```python
from build123d import *

# Parameters (mm, degrees)
ESQUISSE1_W             = 22.5
ESQUISSE1_H             = 80
BOSS_EXTRU_1_DEPTH      = 3
ESQUISSE2_W             = 3
ESQUISSE2_H             = 80
BOSS_EXTRU_2_DEPTH      = 111.5
ESQUISSE3_W             = 22.5
ESQUISSE3_H             = 80
BOSS_EXTRU_3_DEPTH      = 3
ESQUISSE4_R             = 5.25
ENL_V_MAT_EXTRU_1_DEPTH = 2.2
ENL_V_START             = -1.8
ENL_V_MAT_EXTRU_2_DEPTH = 1.2
ENL_V_START_2           = -2.2
ESQUISSE6_R             = 5.25
ENL_V_MAT_EXTRU_3_DEPTH = 2.2
BOSS_EXTRU_4_DEPTH      = 1
ESQUISSE8_R             = 1.6
ENL_V_MAT_EXTRU_4_DEPTH = 4
CONG_2_R                = 1


with BuildPart() as part:
    # Esquisse1 → Boss.-Extru.1 (new body)
    with BuildSketch(Plane.XY):
        with Locations((11.25, 40)):
            Rectangle(ESQUISSE1_W, ESQUISSE1_H)
    extrude(amount=BOSS_EXTRU_1_DEPTH)

    # Esquisse2 → Boss.-Extru.2 (add)
    with BuildSketch(Plane.XY.offset(3)):
        with Locations((1.5, 40)):
            Rectangle(ESQUISSE2_W, ESQUISSE2_H)
    extrude(amount=BOSS_EXTRU_2_DEPTH)

    # Esquisse3 → Boss.-Extru.3 (add)
    with BuildSketch(Plane.XY.offset(114.5)):
        with Locations((11.25, 40)):
            Rectangle(ESQUISSE3_W, ESQUISSE3_H)
    extrude(amount=BOSS_EXTRU_3_DEPTH)

    # Esquisse4 → Enlèv. mat.-Extru.1 (cut)
    with BuildSketch(Plane(origin=(0, 0, 0), x_dir=(-1, 0, 0), z_dir=(0, 0, -1))):
        with Locations((-11.25, 10.15)):
            Circle(ESQUISSE4_R)
        with Locations((-11.25, 70.15)):
            Circle(ESQUISSE4_R)
    extrude(amount=-ENL_V_MAT_EXTRU_1_DEPTH, mode=Mode.SUBTRACT)

    # Esquisse5 → Enlèv. mat.-Extru.2 (cut)
    with BuildSketch(Plane.XY.offset(3).offset(ENL_V_START)):
        Polygon((4.5, 37.75), (9, 37.75), (9, 33.25), (13.5, 33.25), (13.5, 37.75), (18, 37.75), (18, 42.25), (13.5, 42.25), (13.5, 46.75), (9, 46.75), (9, 42.25), (4.5, 42.25), align=None)
    extrude(amount=-ENL_V_MAT_EXTRU_2_DEPTH, mode=Mode.SUBTRACT)

    # Esquisse6 → Enlèv. mat.-Extru.3 (cut)
    with BuildSketch(Plane.XY.offset(117.5).offset(ENL_V_START_2)):
        with Locations(Location((11.25, 10.15, 0), (0, 0, 180))):
            Circle(ESQUISSE6_R)
        with Locations(Location((11.25, 70.15, 0), (0, 0, 180))):
            Circle(ESQUISSE6_R)
    extrude(amount=ENL_V_MAT_EXTRU_3_DEPTH, mode=Mode.SUBTRACT)

    # Esquisse7 → Boss.-Extru.4 (add)
    with BuildSketch(Plane.XY.offset(117.5)):
        Polygon((5.25, 42), (9.25, 42), (9.25, 46), (13.25, 46), (13.25, 42), (17.25, 42), (17.25, 38), (13.25, 38), (13.25, 34), (9.25, 34), (9.25, 38), (5.25, 38), align=None)
    extrude(amount=BOSS_EXTRU_4_DEPTH)

    # Esquisse8 → Enlèv. mat.-Extru.4 (cut)
    with BuildSketch(Plane.ZY):
        with Locations((35.1, 76)):
            Circle(ESQUISSE8_R)
        with Locations((35.1, 66)):
            Circle(ESQUISSE8_R)
        with Locations((17.1, 76)):
            Circle(ESQUISSE8_R)
        with Locations((17.1, 66)):
            Circle(ESQUISSE8_R)
        with Locations((17.1, 4)):
            Circle(ESQUISSE8_R)
        with Locations((17.1, 14)):
            Circle(ESQUISSE8_R)
        with Locations((35.1, 14)):
            Circle(ESQUISSE8_R)
        with Locations((35.1, 4)):
            Circle(ESQUISSE8_R)
        with Locations((83.1, 76)):
            Circle(ESQUISSE8_R)
        with Locations((83.1, 66)):
            Circle(ESQUISSE8_R)
        with Locations((101.1, 76)):
            Circle(ESQUISSE8_R)
        with Locations((101.1, 66)):
            Circle(ESQUISSE8_R)
        with Locations((83.1, 14)):
            Circle(ESQUISSE8_R)
        with Locations((83.1, 4)):
            Circle(ESQUISSE8_R)
        with Locations((101.1, 4)):
            Circle(ESQUISSE8_R)
        with Locations((101.1, 14)):
            Circle(ESQUISSE8_R)
    extrude(amount=-ENL_V_MAT_EXTRU_4_DEPTH, mode=Mode.SUBTRACT)

    # Congé2
    cong_2_edges = [part.edges().sort_by_distance(p)[0] for p in [
        (11.25, 46, 118.5),
        (9.25, 44, 118.5),
        (13.25, 44, 118.5),
        (15.25, 42, 118.5),
        (17.25, 40, 118.5),
        (15.25, 38, 118.5),
        (13.25, 36, 118.5),
        (9.25, 36, 118.5),
        (7.25, 38, 118.5),
        (7.25, 42, 118.5),
        (5.25, 40, 118.5),
        (11.25, 34, 118.5),
    ]]
    fillet(cong_2_edges, radius=CONG_2_R - 0.0001)  # a hair under: the kernel refuses the full size


solid = part.part
```
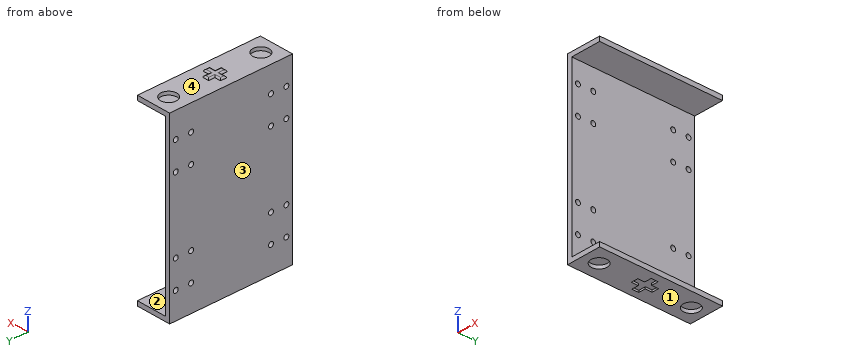
Work out the finished part from the listing and answer in its coordinate system (mm). Face numbers are marked on the shaded views. Give positions to 0.01 mm unless a question says otherwise; leave off trailing zeros. Order: outer loops, then holes, each group sorted by start corner. A loop starts at its lowest first (then second) coordinate and runs counter-clockwise, first axis right, second up.
1. Section A-A, the plane z = 35.1 is taken. Determine the outline of the cut face in (x, y), and give its area (3 significant figures).
Result sheet:
outline: (0, 0) - (3, 0) - (3, 2.4) - (0, 2.4) - close; (0, 5.6) - (3, 5.6) - (3, 12.4) - (0, 12.4) - close; (0, 15.6) - (3, 15.6) - (3, 64.4) - (0, 64.4) - close; (0, 67.6) - (3, 67.6) - (3, 74.4) - (0, 74.4) - close; (0, 77.6) - (3, 77.6) - (3, 80) - (0, 80) - close
area: 202 mm2
2. The mould has two halves that part along Z. Classify the marked faces 1, 2, 3 and 4: released by +Z, released by -Z, zero draft, split by the parting line, or undercut.
Result sheet:
face 1: released by -Z
face 2: undercut
face 3: zero draft
face 4: released by +Z
3. Section C-C, the plane y = 10.15 is taken. Determine the outline of the cut face in (x, z), and give its area (3 significant figures).
Result sheet:
outline: (0, 0) - (6, 0) - (6, 2.2) - (16.5, 2.2) - (16.5, 0) - (22.5, 0) - (22.5, 3) - (3, 3) - (3, 114.5) - (22.5, 114.5) - (22.5, 117.5) - (16.5, 117.5) - (16.5, 115.3) - (6, 115.3) - (6, 117.5) - (0, 117.5) - close
area: 423 mm2
4. Each of these flat-tipped pins is pushed along its axis until it touches: P1, Ø10, axis at x = 12.5, z = 86, coming from the -Y side; P2, Ø12, axis at y = 18, z = 49.5, coming from the +X side; P3, Ø6, axis at x = 15, y = 24.5, coming from the +Z side. Where does it stop, or does it pass through?
Result sheet:
P1: passes through
P2: stops at x = 3
P3: stops at z = 117.5
5. Section B-B, the plane x = 20 is taken. Determine the outline of the cut face in (y, z).
Result sheet:
outline: (0, 0) - (80, 0) - (80, 3) - (0, 3) - close; (0, 114.5) - (80, 114.5) - (80, 117.5) - (0, 117.5) - close
6. Section D-D, the plane y = 32 is taken. Determine the outline of the cut face in (x, z).
Result sheet:
outline: (0, 0) - (22.5, 0) - (22.5, 3) - (3, 3) - (3, 114.5) - (22.5, 114.5) - (22.5, 117.5) - (0, 117.5) - close
7. Straight lines are drawn through the part: L1, parallel to Z at x = 0.8, y = 76; L2, parallel to Y at x = 11.25, z = 116.4; L3, parallel to Y at x = 1.85, z = 101.1. For each, find the intervals that lie inside material, in ascending order.
Result sheet:
L1: z = 0 to 15.5, 18.7 to 33.5, 36.7 to 81.5, 84.7 to 99.5, 102.7 to 117.5
L2: y = 0 to 4.9, 15.4 to 64.9, 75.4 to 80
L3: y = 0 to 2.4, 5.6 to 12.4, 15.6 to 64.4, 67.6 to 74.4, 77.6 to 80
